```python
from build123d import *

# Parameters (mm, degrees)
SKETCH_1_R          = 2
EXTRUDE_1_DEPTH     = 20
SKETCH_2_W          = 18
SKETCH_2_H          = 18
CUT_EXTRUDE_1_DEPTH = 124.162075769


with BuildPart() as part:
    # 草图1 → 凸台-拉伸1 (new body)
    with BuildSketch(Plane.XY):
        Polygon((-47.722320689, -23.749341584), (-37.722320689, -41.06984966), (57.484792643, 13.898002851), (57.484792643, 36.992013619), align=None)
        with Locations((43.880219689, 17.590404378)):
            Circle(SKETCH_1_R, mode=Mode.SUBTRACT)
        with Locations((9.239203538, -2.409595622)):
            Circle(SKETCH_1_R, mode=Mode.SUBTRACT)
        with Locations((0.5789495, -7.409595622)):
            Circle(SKETCH_1_R, mode=Mode.SUBTRACT)
        with Locations((-16.712437168, -17.458303329)):
            Circle(SKETCH_1_R, mode=Mode.SUBTRACT)
        with Locations((-34.032945243, -27.458303329)):
            Circle(SKETCH_1_R, mode=Mode.SUBTRACT)
    extrude(amount=EXTRUDE_1_DEPTH)

    # 草图2 → 切除-拉伸1 (cut, through all)
    with BuildSketch(Plane(origin=(-46.075507084, -26.601706418, 0), x_dir=(0, 0, 1), z_dir=(-0.8660254037844416, -0.49999999999999517, 0))):
        with Locations((10, -6.70637279)):
            Rectangle(SKETCH_2_W, SKETCH_2_H)
    extrude(amount=-CUT_EXTRUDE_1_DEPTH, mode=Mode.SUBTRACT)


solid = part.part
```
Could you check a few things on this model? Use its own coordinates, in mm. A direction names the side the tool comes from. Round coordinates to 2 decimals unless told otherwise and drop trailing zeros. Loops run counter-clockwise (first coordinate to the right, second up) from the corner with the lowest first, then second, coordinate; pieces in that order, holes last. Notation, with made-up numbers: M 0,-11 L 13,-11 A7 cw 13,-1 Z; hole C -35.75,86.5 d3. An arc over 180 degrees is marked long. Answer as CSV lines item,"result".
1) Imagine slicing it at A-A on z = 10. List the corners of the cut face in (x, y) for me, and give its area (3 significant figures).
From the geometry:
outline,"M -47.72,-23.75 L -47.22,-24.62 L 57.48,35.84 L 57.48,36.99 Z; M -38.22,-40.2 L -37.72,-41.07 L 57.48,13.9 L 57.48,15.05 Z"
area,"231 mm^2"
2) For pin 1 Ø1.5 at (x, z) = (35, 8) entering from +Y; pin 2 Ø1.5 at (x, z) = (-36, 17.5) entering from -Y; pin 3 Ø4 at (x, z) = (7, 10.5) entering from -Y, each with a flat end and sliding along its axis, tell me the tip position at first contact or that it passes through.
From the geometry:
pin 1,"y = 24.44"
pin 2,"y = -40.51"
pin 3,"y = -16.4"
3) We'd pull the mould along X, two halves only. Please class faces 1 (the flat face through (4.4, 5.19, 9.87)), 2 (the flat face through (-43.116, -31.728, 19.583)), 3 (the flat face through (9, -5, 20)): released by +X, released by -X, zero draft, split by the parting line, or undercut.
From the geometry:
face 1,"undercut"
face 2,"released by -X"
face 3,"zero draft"
4) Imagine slicing it at D-D on x = -41. List the corners of the cut face in (y, z) for me.
From the geometry:
outline,"M -35.39,0 L -19.87,0 L -19.87,20 L -35.39,20 L -35.39,19 L -21.02,19 L -21.02,1 L -35.39,1 Z"
5) Which directions (+Z, -Z, +X, -X, +Y, -Y) give clear straight access to the entire face, cutting with the end or side of a thin tool? Please do faces 4 (the flat face through (8.961, -12.962, 9.874)), 5 (the flat face through (9.215, -13.971, 9.86)).
From the geometry:
face 4,"none"
face 5,"+Z, -Z, +X, -Y"
6) Imagine slicing it at B-B on x = 13. List the corners of the cut face in (y, z) for me.
From the geometry:
outline,"M -11.79,0 L 11.31,0 L 11.31,20 L -11.79,20 Z; hole M -10.63,1 L 10.15,1 L 10.15,19 L -10.63,19 Z"
7) If I drill on probe 1 along Z at (x, y) = (5.5, -1); probe 2 along X at (y, z) = (5.5, 4); probe 3 along Y at (x, z) = (-5, 15), over which ranges is the centre line in solid material (lowest first)?
From the geometry:
probe 1,"0 to 1, 19 to 20"
probe 2,"2.94 to 4.94, 40.94 to 42.94"
probe 3,"-22.18 to -21.02, -0.24 to 0.92"
8) Imagine slicing it at C-C on y = 32. List the corners of the cut face in (x, z) for me, and give its area (3 significant figures).
From the geometry:
outline,"M 48.84,0 L 57.48,0 L 57.48,1 L 50.84,1 L 50.84,19 L 57.48,19 L 57.48,20 L 48.84,20 Z"
area,"53.3 mm^2"
